Autodesk Fusion 360 part; units mm, degrees
sketch "Sketch1" plane through (0, 0, 0) normal (0, 0, 1) x (1, 0, 0)
  line L0 (0, 0) -> (40, 0)
  line L1 (40, 0) -> (40, 96)
  line L2 (40, 96) -> (0, 96)
  line L3 (0, 96) -> (0, 0)
  line L4 (20, 0) -> (20, 15)
  line L5 (20, 96) -> (20, 81)
  circle A0 centre (20, 81) radius 2.65
  circle A1 centre (20, 15) radius 2.65
  dimension "d1" = 40
  dimension "d2" = 96
  dimension "d3" = 15
  dimension "d4" = 5.3
  dimension "d5" = 5.3
extrude "Extrude1" add sketch "Sketch1" along normal blind 5
sketch "Sketch2" plane through (0, 0, 5) normal (0, 0, 1) x (-1, 0, 0)
  circle A0 centre (-20, -15) radius 2.65
  circle A1 centre (-20, -81) radius 2.65
  line L0 (0, -96) -> (0, 0)
  line L1 (0, 0) -> (-40, 0)
  line L2 (-40, 0) -> (-40, -96)
  line L3 (-40, -96) -> (0, -96)
  line L4 (0, -48) -> (-40, -48)
  line L5 (-20, -46.5) -> (-20, -1.5)
  line L6 (-20, -34) -> (-30, -34)
  line L7 (-30, -34) -> (-30, -14)
  line L8 (-30, -14) -> (-10, -14)
  line L9 (-10, -14) -> (-10, -34)
  line L10 (-10, -34) -> (-20, -34)
  line L11 (-20, -49.5) -> (-20, -94.5)
  line L12 (-20, -62) -> (-30, -62)
  line L13 (-30, -62) -> (-30, -82)
  line L14 (-30, -82) -> (-10, -82)
  line L15 (-10, -82) -> (-10, -62)
  line L16 (-10, -62) -> (-20, -62)
  circle A2 centre (-30, -14) radius 1.55
  circle A3 centre (-10, -14) radius 1.55
  circle A4 centre (-10, -34) radius 1.55
  circle A5 centre (-30, -34) radius 1.55
  circle A6 centre (-30, -62) radius 1.55
  circle A7 centre (-10, -62) radius 1.55
  circle A8 centre (-10, -82) radius 1.55
  circle A9 centre (-30, -82) radius 1.55
  dimension "d12" = 45
  dimension "d15" = 45
  dimension "d16" = 3.1
  dimension "d17" = 3.1
  dimension "d18" = 3.1
  dimension "d19" = 3.1
  dimension "d20" = 3.1
  dimension "d21" = 3.1
  dimension "d22" = 3.1
  dimension "d23" = 3.1
extrude "Extrude2" cut sketch "Sketch2" against normal blind 5 contours L8 L9 A3 | L8 L9 A3 | L7 L8 A2 | L7 L8 A2 | L6 L7 A5 | L6 L7 A5 | L9 L10 A4 | L9 L10 A4 | L14 L15 A8 | L14 L15 A8 | L13 L14 A9 | L13 L14 A9 | L12 L13 A6 | L12 L13 A6 | L15 L16 A7 | L15 L16 A7
sketch "Sketch3" plane through (0, 0, 5) normal (0, 0, 1) x (-1, 0, 0)
  circle A0 centre (-30, -34) radius 1.55
  circle A1 centre (-10, -82) radius 1.55
  circle A2 centre (-10, -62) radius 1.55
  circle A3 centre (-30, -14) radius 1.55
  circle A4 centre (-10, -34) radius 1.55
  circle A5 centre (-30, -82) radius 1.55
  circle A6 centre (-10, -14) radius 1.55
  circle A7 centre (-30, -62) radius 1.55
  circle A8 centre (-20, -15) radius 2.65
  circle A9 centre (-20, -81) radius 2.65
  line L0 (0, -96) -> (0, 0)
  line L1 (0, 0) -> (-40, 0)
  line L2 (-40, 0) -> (-40, -96)
  line L3 (-40, -96) -> (0, -96)
  circle A10 centre (-20, -15) radius 2.65
  circle A11 centre (-20, -81) radius 2.65
extrude "Extrude3" add sketch "Sketch3" against normal blind 5 contours A8 A10 | A9 A11
sketch "Sketch4" plane through (0, 0, 0) normal (0, 0, 1) x (1, 0, 0)
  line L0 (-10, 0) -> (-10, 30)
  line L1 (-10, 30) -> (0, 30)
  line L2 (-5, 0) -> (-5, 15)
  circle A0 centre (-5, 15) radius 2.6
  line L3 (40, 0) -> (50, 0)
  line L4 (50, 0) -> (50, 30)
  line L5 (50, 30) -> (40, 30)
  line L6 (40, 30) -> (45, 15)
  circle A1 centre (45, 15) radius 2.6
  line L7 (40, 96) -> (50, 96)
  line L8 (50, 96) -> (50, 66)
  line L9 (50, 66) -> (40, 66)
  line L10 (40, 66) -> (45, 80)
  circle A2 centre (45, 80) radius 2.6
  line L11 (0, 96) -> (-10, 96)
  line L12 (-10, 96) -> (-10, 66)
  line L13 (-10, 66) -> (0, 66)
  line L14 (0, 66) -> (-5, 81)
  circle A3 centre (-5, 81) radius 2.6
  line L15 (-10, 0) -> (-9, 0)
  line L16 (-9, 0) -> (0, 0)
  line L17 (0, 0) -> (0, 30)
  line L18 (40, 30) -> (40, 0)
  line L19 (0, 66) -> (0, 96)
  line L20 (40, 96) -> (40, 66)
  dimension "d28" = 5.2
  dimension "d29" = 5.2
  dimension "d30" = 5.2
  dimension "d31" = 5.2
extrude "Extrude4" add sketch "Sketch4" along normal blind 5
chamfer "Chamfer1" distance 10 angle 45 1 edges at (-10, 0, 2.5)
chamfer "Chamfer2" distance 10 angle 45 1 edges at (50, 0, 2.5)
chamfer "Chamfer3" distance 10 angle 45 1 edges at (-10, 96, 2.5)
chamfer "Chamfer4" distance 10 angle 45 1 edges at (50, 96, 2.5)
sketch "Sketch5" plane through (0, 0, 5) normal (0, 0, 1) x (-1, 0, 0)
  circle A0 centre (-45, -80) radius 2.6
  circle A1 centre (-45, -15) radius 2.6
  circle A2 centre (5, -81) radius 2.6
  circle A3 centre (5, -15) radius 2.6
  circle A4 centre (-30, -34) radius 1.55
  circle A5 centre (-10, -82) radius 1.55
  circle A6 centre (-10, -62) radius 1.55
  circle A7 centre (-30, -14) radius 1.55
  circle A8 centre (-10, -34) radius 1.55
  circle A9 centre (-30, -82) radius 1.55
  circle A10 centre (-10, -14) radius 1.55
  circle A11 centre (-30, -62) radius 1.55
  line L0 (-50, -86) -> (-40, -96)
  line L1 (-40, -96) -> (0, -96)
  line L2 (0, -96) -> (10, -86)
  line L3 (10, -86) -> (10, -66)
  line L4 (10, -66) -> (0, -66)
  line L5 (0, -66) -> (0, -30)
  line L6 (0, -30) -> (10, -30)
  line L7 (10, -30) -> (10, -10)
  line L8 (10, -10) -> (0, 0)
  line L9 (0, 0) -> (-40, 0)
  line L10 (-40, 0) -> (-50, -10)
  line L11 (-50, -10) -> (-50, -30)
  line L12 (-50, -30) -> (-40, -30)
  line L13 (-40, -30) -> (-40, -66)
  line L14 (-40, -66) -> (-50, -66)
  line L15 (-50, -66) -> (-50, -86)
  line L16 (-10, -62) -> (-30, -82)
  line L17 (-10, -14) -> (-30, -34)
  circle A12 centre (-20, -24) radius 7
  circle A13 centre (-20, -72) radius 7
  dimension "d38" = 14
  dimension "d39" = 14
extrude "Extrude5" cut sketch "Sketch5" against normal blind 5 contours L17 A12 | L17 A12 | L16 A13 | L16 A13
sketch "Sketch6" plane through (0, 0, 5) normal (0, 0, 1) x (-1, 0, 0)
  circle A0 centre (-20, -24) radius 7
  circle A1 centre (-20, -72) radius 7
  circle A2 centre (-45, -80) radius 2.6
  circle A3 centre (-45, -15) radius 2.6
  circle A4 centre (5, -81) radius 2.6
  circle A5 centre (5, -15) radius 2.6
  circle A6 centre (-30, -34) radius 1.55
  circle A7 centre (-10, -82) radius 1.55
  circle A8 centre (-10, -62) radius 1.55
  circle A9 centre (-30, -14) radius 1.55
  circle A10 centre (-10, -34) radius 1.55
  circle A11 centre (-30, -82) radius 1.55
  circle A12 centre (-10, -14) radius 1.55
  circle A13 centre (-30, -62) radius 1.55
  line L0 (-50, -86) -> (-40, -96)
  line L1 (-40, -96) -> (0, -96)
  line L2 (0, -96) -> (10, -86)
  line L3 (10, -86) -> (10, -66)
  line L4 (10, -66) -> (0, -66)
  line L5 (0, -66) -> (0, -30)
  line L6 (0, -30) -> (10, -30)
  line L7 (10, -30) -> (10, -10)
  line L8 (10, -10) -> (0, 0)
  line L9 (0, 0) -> (-40, 0)
  line L10 (-40, 0) -> (-50, -10)
  line L11 (-50, -10) -> (-50, -30)
  line L12 (-50, -30) -> (-40, -30)
  line L13 (-40, -30) -> (-40, -66)
  line L14 (-40, -66) -> (-50, -66)
  line L15 (-50, -66) -> (-50, -86)
  circle A14 centre (-10, -82) radius 3.25
  circle A15 centre (-30, -82) radius 3.25
  circle A16 centre (-30, -62) radius 3.25
  circle A17 centre (-10, -62) radius 3.25
  circle A18 centre (-10, -34) radius 3.25
  circle A19 centre (-30, -34) radius 3.25
  circle A20 centre (-30, -14) radius 3.25
  circle A21 centre (-10, -14) radius 3.25
  dimension "d42" = 6.5
  dimension "d43" = 6.5
  dimension "d44" = 6.5
  dimension "d45" = 6.5
  dimension "d46" = 6.5
  dimension "d47" = 6.5
  dimension "d48" = 6.5
  dimension "d49" = 6.5
extrude "Extrude6" cut sketch "Sketch6" against normal blind 3.5 contours A14 | A15 | A16 | A17 | A18 | A19 | A20 | A21
Build history of the part. All positions in model axes, mm. A direction names the side the tool comes from. Coordinates: 2 decimals unless noted, no trailing zeros. Order: outer loops, then holes, each group sorted by start corner. A loop starts at its lowest first (then second) coordinate and runs counter-clockwise, first axis right, second up.
Item 1: Saw through at C-C on y = 24. List the corners of the cut face in (x, z).
Filled in:
outline: (-10, 0) - (13, 0) - (13, 5) - (-10, 5) - close; (27, 0) - (50, 0) - (50, 5) - (27, 5) - close
Item 2: Tool access for faces 1 (the cylindrical face through (13.247, 13.857, 3.274)), 2 (the flat face through (45, 30, 2)), 3 (the flat face through (-5, 5, 3)), 4 (the flat face through (-5, 30, 2)): list every direction of +Z, -Z, +X, -X, +Y, -Y with a clear straight run to the whole face (end or side of a thin tool).
Filled in:
face 1: +Z
face 2: +Z, -Z, +X
face 3: +Z, -Z, -X, -Y
face 4: +Z, -Z, -X
Item 3: Saw through at D-D on x = 20. List the corners of the cut face in (y, z).
Filled in:
outline: (0, 0) - (17, 0) - (17, 5) - (0, 5) - close; (31, 0) - (65, 0) - (65, 5) - (31, 5) - close; (79, 0) - (96, 0) - (96, 5) - (79, 5) - close
Item 4: Mould opens along Y. For faces 5 (the cylindrical face through (30.202, 60.463, 0.761)), 6 (the flat face through (45, 5, 3)), 7 (the flat face through (50, 76, 2)) say: released by +Y, released by -Y, zero draft, split by the parting line, or undercut.
Filled in:
face 5: undercut
face 6: released by -Y
face 7: zero draft
Item 5: Saw through at A-A on z = 3.65. State how many separate pieces and enclosed holes the cut face has, then the cut area to 3 significant figures.
Filled in:
separate pieces: 1
enclosed holes: 14
area: 4,180 mm2
Item 6: Drill centre lines: L1, parallel to X at y = 34, z = 0.6; L2, parallel to Y at x = 10, z = 1.2; L3, parallel to Y at x = 10, z = 3.4. Where is each one in solid material? Low to high.
Filled in:
L1: x = 0 to 8.45, 11.55 to 28.45, 31.55 to 40
L2: y = 0 to 12.45, 15.55 to 32.45, 35.55 to 60.45, 63.55 to 80.45, 83.55 to 96
L3: y = 0 to 10.75, 17.25 to 30.75, 37.25 to 58.75, 65.25 to 78.75, 85.25 to 96
Item 7: Saw through at B-B on x = 45. List the corners of the cut face in (y, z), then the cut area to 3 significant figures.
Filled in:
outline: (5, 0) - (12.4, 0) - (12.4, 5) - (5, 5) - close; (17.6, 0) - (30, 0) - (30, 5) - (17.6, 5) - close; (66, 0) - (77.4, 0) - (77.4, 5) - (66, 5) - close; (82.6, 0) - (91, 0) - (91, 5) - (82.6, 5) - close
area: 198 mm2
Item 8: Drop flat-ended pins along their axis: pin 1 Ø3 at (y, z) = (40, 2) entering from +X; pin 2 Ø1.5 at (x, z) = (43.5, 1.5) entering from +Y; pin 3 Ø2 at (x, y) = (29.5, 62.5) entering from +Z; pin 4 Ø11 at (x, y) = (20, 24) entering from +Z. Give the stop position or say it passes through.
Filled in:
pin 1: stops at x = 40
pin 2: stops at y = 93.25
pin 3: stops at z = 1.5
pin 4: passes through
